For this review, use the dimensioned drawing (mm, ordinates from the lowest corner) and the shaded views. Give positions to 0.01 mm unless a question says otherwise; leave off trailing zeros. Order: outer loops, then holes, each group sorted by start corner. A loop starts at its lowest first (then second) coordinate and runs counter-clockwise, first axis right, second up. Notation, with made-up numbers: (-25.5, -35) - (30.5, -35) arc R29 cw to (30.5, -3) - close; hole circle Ø10 at (-36, 60). An arc over 180 degrees is marked (long way). Answer as CSV lines item,"result". Start each with the question number.
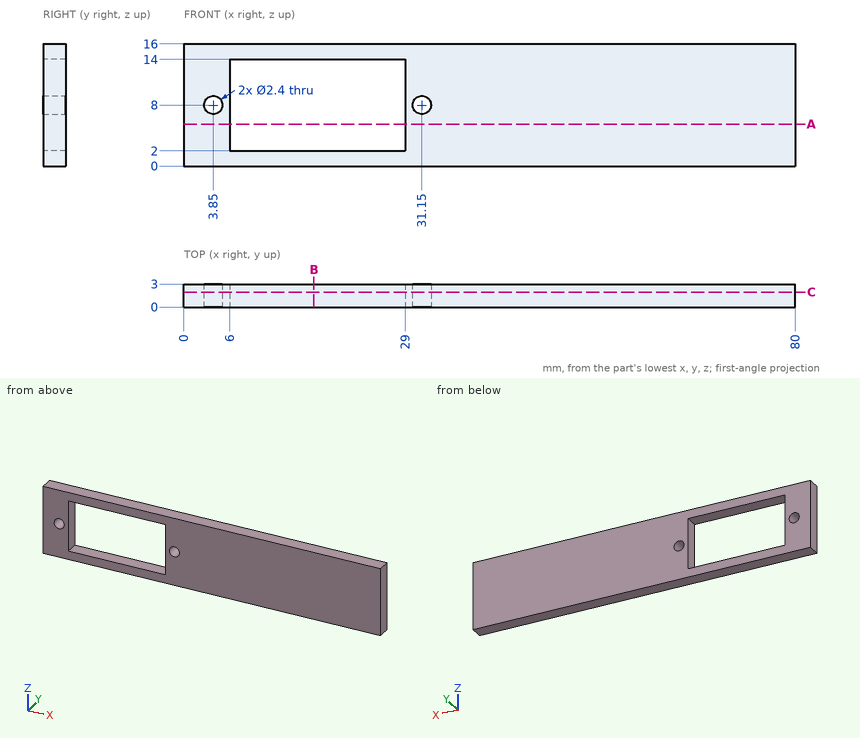
Item 1: Take a section at B-B on x = 17. Write out the cut boundary in (y, z).
Item 2: Take a section at C-C on y = 1.95. Write out the cut boundary in (x, z), and give its area (3 significant figures).
Item 3: For line 1 along X through (y, z) = (2.25, 8); line 2 along Z through (x, y) = (13.5, 0.35); line 3 along Z through (x, y) = (31.15, 1.4), list the stretches that pass through material, from the lowest coordinate up.
Item 4: Clearance check with a flat-ended pin moving along its axis: pin 1 (1.4 mm diameter, centred on x = 3.85, z = 8, fed in from -Y). State where the tip first meets the part, or that it passes through.
Item 5: Take a section at A-A on z = 5.5. Write out the cut boundary in (x, y).
Data:
1,outline,"(0, 0) - (3, 0) - (3, 2) - (0, 2) - close; (0, 14) - (3, 14) - (3, 16) - (0, 16) - close"
2,outline,"(0, 0) - (80, 0) - (80, 16) - (0, 16) - close; hole circle Ø2.4 at (3.85, 8); hole (6, 2) - (29, 2) - (29, 14) - (6, 14) - close; hole circle Ø2.4 at (31.15, 8)"
2,area,"995 mm^2"
3,line 1,"x = 0 to 2.65, 5.05 to 6, 29 to 29.95, 32.35 to 80"
3,line 2,"z = 0 to 2, 14 to 16"
3,line 3,"z = 0 to 6.8, 9.2 to 16"
4,pin 1,"passes through"
5,outline,"(0, 0) - (6, 0) - (6, 3) - (0, 3) - close; (29, 0) - (80, 0) - (80, 3) - (29, 3) - close"
